Part model, mm, in its own coordinate system. A direction names the side the tool comes from. Give positions to 0.01 mm unless a question says otherwise; leave off trailing zeros. Write each loop counter-clockwise with the first axis right and the second up, starting at its lowest first coordinate (ties: lowest second). Pieces come first, ordered by that corner, then holes.
```python
from build123d import *

# Parameters (mm, degrees)
BASE_FLANGE1_DEPTH      = 111.125
SKETCH16_R              = 14.2875
SKETCH16_R_2            = 2.5146
CUT_EXTRUDE1_DEPTH      = 172.596927784
CUT_EXTRUDE2_DEPTH      = 2.54
CUT_EXTRUDE2_DEPTH_BACK = 172.596927784


# Read off the part's stored shape, not the designer's step: Base-Flange1
with BuildPart() as part:
    # Base-Flange1 outline → Base-Flange1 (new body)
    with BuildSketch(Plane.XY):
        with BuildLine():
            Line((60.325, -3.937), (60.325, -114.3))
            Line((60.325, -114.3), (63.5, -114.3))
            Line((63.5, -114.3), (63.5, -3.937))
            ThreePointArc((63.5, -3.937), (62.346879398, -1.153120602), (59.563, 0))
            Line((59.563, 0), (0, 0))
            Line((0, 0), (0, -3.175))
            Line((0, -3.175), (59.563, -3.175))
            ThreePointArc((59.563, -3.175), (60.101815367, -3.398184633), (60.325, -3.937))
        make_face()
    extrude(amount=BASE_FLANGE1_DEPTH)

    # Sketch16 → Cut-Extrude1 (cut, through all)
    with BuildSketch(Plane(origin=(63.5, 0, 0), x_dir=(0, 0, -1), z_dir=(1, 0, 0))):
        with Locations((-79.375, -80.9625)):
            Circle(SKETCH16_R)
        with Locations((-15.875, -39.6875)):
            Circle(SKETCH16_R)
        with Locations((-53.975, -15.875)):
            Circle(SKETCH16_R_2)
        with Locations((-53.975, -34.925)):
            Circle(SKETCH16_R_2)
        with Locations((-73.025, -15.875)):
            Circle(SKETCH16_R_2)
        with Locations((-73.025, -34.925)):
            Circle(SKETCH16_R_2)
        with Locations((-92.075, -15.875)):
            Circle(SKETCH16_R_2)
        with Locations((-92.075, -34.925)):
            Circle(SKETCH16_R_2)
        Polygon((0, -44.774825848), (-52.3875, -114.3), (0, -114.3), align=None)
    extrude(amount=-CUT_EXTRUDE1_DEPTH, mode=Mode.SUBTRACT)

    # Sketch17 → Cut-Extrude2 (cut, two sides: drawn at the far end of the back side and taken through both)
    with BuildSketch(Plane(origin=(0, 0, 0), x_dir=(1, 0, 0), z_dir=(0, 1, 0)).offset(-CUT_EXTRUDE2_DEPTH_BACK)):
        Polygon((-184.195113126, 135.751553806), (0, -50.8), (59.563, -111.125), (243.758113126, -297.676553806), (-129.344994485, -666.066780058), (-557.298220737, -232.638672446), align=None)
    extrude(amount=CUT_EXTRUDE2_DEPTH + CUT_EXTRUDE2_DEPTH_BACK, mode=Mode.SUBTRACT)


solid = part.part
```
1) Saw through at D-D, the plane y = -21. Write the cut outline in (x, z) (3 decimals), then the cut area to 3 significant figures.
Answers follow:
outline: (60.325, 0) - (63.5, 0) - (63.5, 111.125) - (60.325, 111.125) - close
area: 353 mm2
2) Two-plate mould, pull along Z, no slides. Class faces 1 (the face through (61.935, -79.051, 25.827)), 2 (the face through (61.93, -32.43, 92.4)), 3 (the face through (60.325, -46, 67)): +Z half, -Z half, draft (parallel to the pull), parting line (faces both ways), or undercut.
Answers follow:
face 1: -Z half
face 2: undercut
face 3: draft
3) Saw through at C-C, the plane z = 59. Write the cut outline in (x, y) (3 decimals).
Answers follow:
outline: (8.096, -3.175) - (59.563, -3.175) arc R0.762 cw to (60.325, -3.937) - (60.325, -114.3) - (63.5, -114.3) - (63.5, -3.937) arc R3.937 ccw to (59.563, 0) - (8.096, 0) - close
4) Pin check, flat tips, straight feed: pin 1 Ø10 at (x, z) = (41.5, 28) entering from -Y (3 decimals); pin 2 Ø4 at (y, z) = (-14.5, 55) entering from +X; pin 3 Ø6 at (y, z) = (-34.925, 53.975) entering from -X (3 decimals). Stop position of each tip, or through.
Answers follow:
pin 1: stops at y = -3.175
pin 2: stops at x = 63.5
pin 3: stops at x = 60.325
5) Saw through at B-B, the plane y = -87. Write the cut outline in (x, z) (3 decimals).
Answers follow:
outline: (60.325, 31.817) - (63.5, 31.817) - (63.5, 66.426) - (60.325, 66.426) - close; (60.325, 92.324) - (63.5, 92.324) - (63.5, 111.125) - (60.325, 111.125) - close
6) 3-axis set-ups, long thin cutter, end or side, ignore diameter. For faces 4 (the face through (61.935, -34.17, 70.627)), 5 (the face through (36, -3.175, 42)): which of +Z, -Z, +X, -X, +Y, -Y reach the whole face in a straight line?
Answers follow:
face 4: +X, -X
face 5: +Z, -Z, -X, -Y
7) Saw through at A-A, the plane z = 81.5. Write the cut outline in (x, y) (3 decimals), then the cut area to 3 significant figures.
Answers follow:
outline: (30.312, -3.175) - (59.563, -3.175) arc R0.762 cw to (60.325, -3.937) - (60.325, -66.834) - (63.5, -66.834) - (63.5, -3.937) arc R3.937 ccw to (59.563, 0) - (30.312, 0) - close; (60.325, -114.3) - (63.5, -114.3) - (63.5, -95.091) - (60.325, -95.091) - close
area: 365 mm2
8) Wall check: L1, parallel to Y at x = 40, z = 21.5 (3 decimals); L2, parallel to X at y = -94, z = 90 (3 decimals); L3, parallel to Y at x = 60, z = 64.5. Give the ranges that are in metal, low to high.
Answers follow:
L1: y = -3.175 to 0
L2: x = 60.325 to 63.5
L3: y = -3.31 to -0.02
